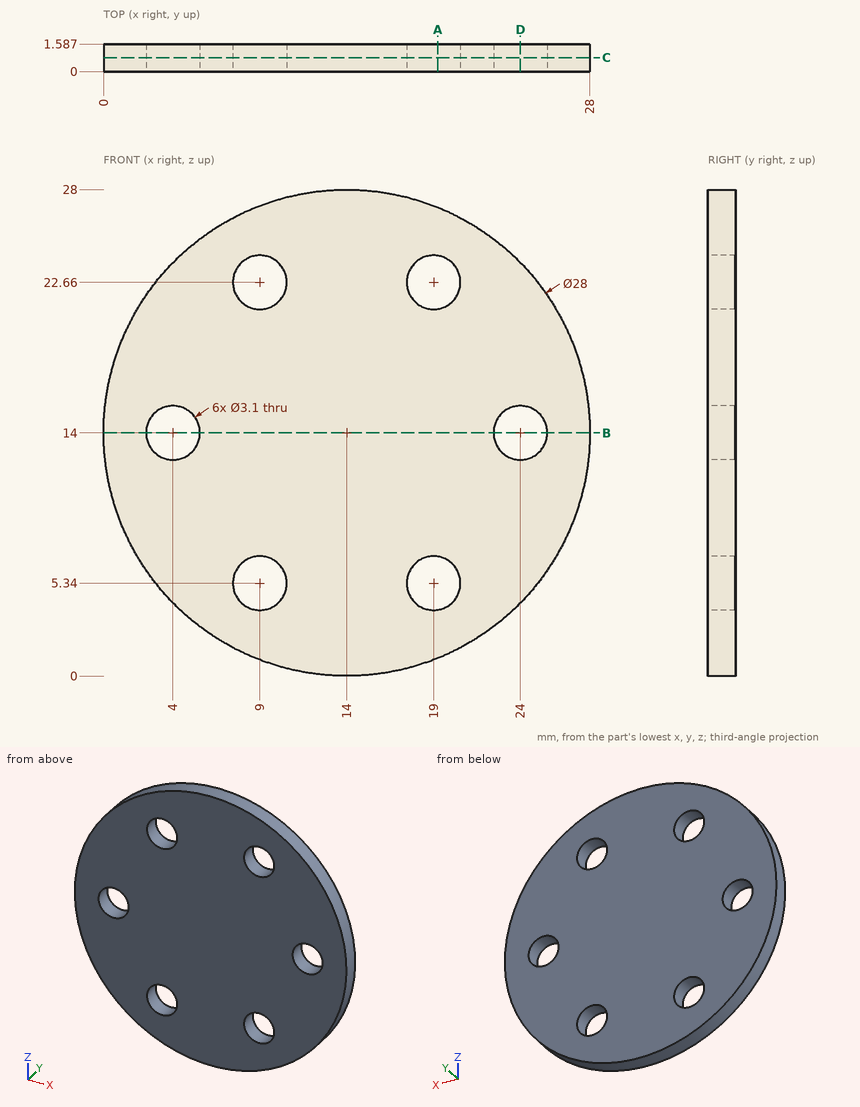
Part print with two shaded views. Sizes in mm from the minimum x, y, z corner. Round coordinates to 2 decimals unless told otherwise and drop trailing zeros. Order: outer loops, then holes, each group sorted by start corner. A loop starts at its lowest first (then second) coordinate and runs counter-clockwise, first axis right, second up. Notation, with made-up numbers: (52.5, 22) -> (77.5, 22) arc R24 ccw to (77.5, 56) -> close; hole circle Ø9 at (-5, 76.25). An arc over 180 degrees is marked (long way). Use one line per item in the form item = value.
Item 1: Cut at B-B, the plane z = 14. Write the cut outline in (x, y).
Returned:
outline = (0, 0) -> (2.45, 0) -> (2.45, 1.59) -> (0, 1.59) -> close; (5.55, 0) -> (22.45, 0) -> (22.45, 1.59) -> (5.55, 1.59) -> close; (25.55, 0) -> (28, 0) -> (28, 1.59) -> (25.55, 1.59) -> close
Item 2: Cut at A-A, the plane x = 19.25. Write the cut outline in (y, z).
Returned:
outline = (0, 1.02) -> (1.59, 1.02) -> (1.59, 3.81) -> (0, 3.81) -> close; (0, 6.87) -> (1.59, 6.87) -> (1.59, 21.13) -> (0, 21.13) -> close; (0, 24.19) -> (1.59, 24.19) -> (1.59, 26.98) -> (0, 26.98) -> close
Item 3: Cut at C-C, the plane y = 0.8. Write the cut outline in (x, z).
Returned:
outline = circle Ø28 at (14, 14); hole circle Ø3.1 at (4, 14); hole circle Ø3.1 at (9, 5.34); hole circle Ø3.1 at (9, 22.66); hole circle Ø3.1 at (19, 5.34); hole circle Ø3.1 at (19, 22.66); hole circle Ø3.1 at (24, 14)
Item 4: Cut at D-D, the plane x = 24. Write the cut outline in (y, z).
Returned:
outline = (0, 4.2) -> (1.59, 4.2) -> (1.59, 12.45) -> (0, 12.45) -> close; (0, 15.55) -> (1.59, 15.55) -> (1.59, 23.8) -> (0, 23.8) -> close
Item 5: Drill centre lines: line 1 (X direction, y = 0.45, z = 14); line 2 (Z direction, x = 18.75, y = 1.05); line 3 (X direction, y = 0.1, z = 24) (1 decimal). Where is each one in solid material? Low to high.
Returned:
line_1 = 0 to 2.45, 5.55 to 22.45, 25.55 to 28
line_2 = 0.83 to 3.81, 6.87 to 21.13, 24.19 to 27.17
line_3 = 4.2 to 8.2, 9.8 to 18.2, 19.8 to 23.8
